Check sheet for the modelled part. Datum: model origin and axes. Units: mm. A direction names the side the tool comes from. Round coordinates to 2 decimals unless told otherwise and drop trailing zeros. Loops run counter-clockwise (first coordinate to the right, second up) from the corner with the lowest first, then second, coordinate; pieces in that order, holes last. Notation, with made-up numbers: (-33, 87.5) -> (21, 87.5) arc R9 cw to (21, 100.5) -> close; hole circle Ø6 at (48.25, 62.25). An arc over 180 degrees is marked (long way). One line per item, written item: value. Start each with the question number.
1. Release check for a two-part mould opening along X. For faces 1 (the face through (1, -1, 3)), 2 (the face through (-18, -0.5, 1)) record: +X half, -X half, draft (parallel to the pull), parting line (faces both ways), or undercut.
2. Cross-section at B-B on x = 33. Record the cut outline in (y, z).
3. Cross-section at A-A on y = 6.25. Record the cut outline in (x, z), then the cut area to 3 significant figures.
4. Set-up check for faces 3 (the face through (54, -0.5, 1)), 4 (the face through (28.5, 6, 1)), 5 (the face through (54, -7.5, 1)), 6 (the face through (-34, -10.5, 1)): record each of +Z, -Z, +X, -X, +Y, -Y from which the full face is reachable in a straight line by a thin tool's end or side.
5. Go/stop test with a flat-tipped pin: pin 1 (0.9 mm diameter, centred on x = 56.5, z = 1, fed in from -Y). Record where the tip stops, or that it passes through.
6. Cross-section at C-C on y = -8.75. Record the cut outline in (x, z).
7. Material ranges on L1, parallel to X at y = -10, z = 1.55; L2, parallel to Y at x = -39, z = 0.7; L3, parallel to Y at x = 55.5, z = 1.3, recorded low to high.
8. Cross-section at D-D on z = 2.1. Count the separate pieces of the cut face and the enclosed holes in it, then the cut area to 3 significant figures.
from build123d import *

# Parameters (mm, degrees)
SKETCH2_W           = 10
SKETCH2_H           = 3
BOSS_EXTRUDE2_DEPTH = 3


with BuildPart() as part:
    # Sketch2 → Boss-Extrude2 (new body)
    with BuildSketch(Plane.XY):
        Polygon((-43.5, 7.5), (-28.5, 7.5), (-28.5, 4.5), (-25.5, 4.5), (-25.5, 7.5), (-10.5, 7.5), (-10.5, 4.5), (-7.5, 4.5), (-7.5, 7.5), (7.5, 7.5), (7.5, 4.5), (10.5, 4.5), (10.5, 7.5), (25.5, 7.5), (25.5, 4.5), (28.5, 4.5), (28.5, 7.5), (43.5, 7.5), (43.5, 4.5), (46.5, 4.5), (46.5, 7.5), (61.5, 7.5), (61.5, -7.5), (46.5, -7.5), (46.5, -10.5), (21.5, -10.5), (21.5, -7.5), (10, -7.5), (-10, -7.5), (-21.5, -7.5), (-21.5, -10.5), (-46.5, -10.5), (-46.5, -7.5), (-61.5, -7.5), (-61.5, 7.5), (-46.5, 7.5), (-46.5, 4.5), (-43.5, 4.5), align=None)
        with Locations((-54, 1)):
            Rectangle(SKETCH2_W, SKETCH2_H, mode=Mode.SUBTRACT)
        with Locations((-36, 1)):
            Rectangle(SKETCH2_W, SKETCH2_H, mode=Mode.SUBTRACT)
        with Locations((-18, 1)):
            Rectangle(SKETCH2_W, SKETCH2_H, mode=Mode.SUBTRACT)
        with Locations((0, 1)):
            Rectangle(SKETCH2_W, SKETCH2_H, mode=Mode.SUBTRACT)
        with Locations((18, 1)):
            Rectangle(SKETCH2_W, SKETCH2_H, mode=Mode.SUBTRACT)
        with Locations((36, 1)):
            Rectangle(SKETCH2_W, SKETCH2_H, mode=Mode.SUBTRACT)
        with Locations((54, 1)):
            Rectangle(SKETCH2_W, SKETCH2_H, mode=Mode.SUBTRACT)
    extrude(amount=BOSS_EXTRUDE2_DEPTH)


solid = part.part
Taken from the geometry:
1. face 1: draft
1. face 2: undercut
2. outline: (-10.5, 0) -> (-0.5, 0) -> (-0.5, 3) -> (-10.5, 3) -> close; (2.5, 0) -> (7.5, 0) -> (7.5, 3) -> (2.5, 3) -> close
3. outline: (-61.5, 0) -> (-46.5, 0) -> (-46.5, 3) -> (-61.5, 3) -> close; (-43.5, 0) -> (-28.5, 0) -> (-28.5, 3) -> (-43.5, 3) -> close; (-25.5, 0) -> (-10.5, 0) -> (-10.5, 3) -> (-25.5, 3) -> close; (-7.5, 0) -> (7.5, 0) -> (7.5, 3) -> (-7.5, 3) -> close; (10.5, 0) -> (25.5, 0) -> (25.5, 3) -> (10.5, 3) -> close; (28.5, 0) -> (43.5, 0) -> (43.5, 3) -> (28.5, 3) -> close; (46.5, 0) -> (61.5, 0) -> (61.5, 3) -> (46.5, 3) -> close
3. area: 315 mm2
4. face 3: +Z, -Z
4. face 4: +Z, -Z, +Y
4. face 5: +Z, -Z, +X, -Y
4. face 6: +Z, -Z, +X, -X, -Y
5. pin 1: stops at y = -7.5
6. outline: (-46.5, 0) -> (-21.5, 0) -> (-21.5, 3) -> (-46.5, 3) -> close; (21.5, 0) -> (46.5, 0) -> (46.5, 3) -> (21.5, 3) -> close
7. L1: x = -46.5 to -21.5, 21.5 to 46.5
7. L2: y = -10.5 to -0.5, 2.5 to 7.5
7. L3: y = -7.5 to -0.5, 2.5 to 7.5
8. separate pieces: 1
8. enclosed holes: 7
8. area: 1,730 mm2
